The listing builds one solid part. Answer for the finished solid, in the listing's coordinates (mm). Coordinates: 2 decimals unless noted, no trailing zeros. Loops run counter-clockwise (first coordinate to the right, second up) from the corner with the lowest first, then second, coordinate; pieces in that order, holes last. Notation, with made-up numbers: (-9.5, 26.5) -> (28.5, 26.5) arc R20 cw to (28.5, 33.5) -> close; hole circle Ø11 at (88.5, -33). An arc over 180 degrees is marked (long way). Answer in a Markdown table with one row per item.
```python
from build123d import *

# Parameters (mm, degrees)
SKETCH1_R           = 10
SKETCH1_R_2         = 0.5
BOSS_EXTRUDE1_DEPTH = 3


with BuildPart() as part:
    # Sketch1 → Boss-Extrude1 (new body)
    with BuildSketch(Plane.XY):
        Circle(SKETCH1_R)
        with Locations((0, 9)):
            Circle(SKETCH1_R_2, mode=Mode.SUBTRACT)
        Polygon((2, -0.866025404), (3.5, -1.732050808), (5, -0.866025404), (5, 0.866025404), (3.5, 1.732050808), (2, 0.866025404), align=None, mode=Mode.SUBTRACT)
        Polygon((-1.75, 1.267949192), (-0.25, 2.133974596), (-0.25, 3.866025404), (-1.75, 4.732050808), (-3.25, 3.866025404), (-3.25, 2.133974596), align=None, mode=Mode.SUBTRACT)
        Polygon((-1.5, -0.866025404), (0, -1.732050808), (1.5, -0.866025404), (1.5, 0.866025404), (0, 1.732050808), (-1.5, 0.866025404), align=None, mode=Mode.SUBTRACT)
        Polygon((5.5, -0.866025404), (7, -1.732050808), (8.5, -0.866025404), (8.5, 0.866025404), (7, 1.732050808), (5.5, 0.866025404), align=None, mode=Mode.SUBTRACT)
        Polygon((-5.5, 0.866025404), (-5.5, -0.866025404), (-7, -1.732050808), (-8.5, -0.866025404), (-8.5, 0.866025404), (-7, 1.732050808), align=None, mode=Mode.SUBTRACT)
        Polygon((-2, 0.866025404), (-2, -0.866025404), (-3.5, -1.732050808), (-5, -0.866025404), (-5, 0.866025404), (-3.5, 1.732050808), align=None, mode=Mode.SUBTRACT)
        Polygon((1.75, 1.267949192), (3.25, 2.133974596), (3.25, 3.866025404), (1.75, 4.732050808), (0.25, 3.866025404), (0.25, 2.133974596), align=None, mode=Mode.SUBTRACT)
        Polygon((5.25, 1.267949192), (6.75, 2.133974596), (6.75, 3.866025404), (5.25, 4.732050808), (3.75, 3.866025404), (3.75, 2.133974596), align=None, mode=Mode.SUBTRACT)
        Polygon((-0.25, -2.133974596), (-1.75, -1.267949192), (-3.25, -2.133974596), (-3.25, -3.866025404), (-1.75, -4.732050808), (-0.25, -3.866025404), align=None, mode=Mode.SUBTRACT)
        Polygon((3.25, -2.133974596), (1.75, -1.267949192), (0.25, -2.133974596), (0.25, -3.866025404), (1.75, -4.732050808), (3.25, -3.866025404), align=None, mode=Mode.SUBTRACT)
        Polygon((-3.75, -2.133974596), (-5.25, -1.267949192), (-6.75, -2.133974596), (-6.75, -3.866025404), (-5.25, -4.732050808), (-3.75, -3.866025404), align=None, mode=Mode.SUBTRACT)
    extrude(amount=BOSS_EXTRUDE1_DEPTH)


solid = part.part
```
Item 1: Flat-ended cylindrical pins translate along their axes: pin 1 Ø1.4 at (y, z) = (0.5, 1.5) entering from +X; pin 2 Ø1.5 at (x, z) = (-5.5, 2) entering from -Y; pin 3 Ø0.9 at (y, z) = (3, 2) entering from +X; pin 4 Ø0.5 at (y, z) = (3, 2) entering from +X. Find the tip coordinate at first contact, or state that the pin passes through.
Findings below:
| item | result |
|---|---|
| pin 1 | stops at x = 10 |
| pin 2 | stops at y = -8.8 |
| pin 3 | stops at x = 9.67 |
| pin 4 | stops at x = 9.61 |
Item 2: A cutting plane is placed at D-D, the plane y = 9. Determine the outline of the cut face in (x, z), plus the area to 3 significant figures.
Findings below:
| item | result |
|---|---|
| outline | (-4.36, 0) -> (-0.5, 0) -> (-0.5, 3) -> (-4.36, 3) -> close; (0.5, 0) -> (4.36, 0) -> (4.36, 3) -> (0.5, 3) -> close |
| area | 23.2 mm2 |
Item 3: A cutting plane is placed at A-A, the plane y = 0. Determine the outline of the cut face in (x, z).
Findings below:
| item | result |
|---|---|
| outline | (-10, 0) -> (-8.5, 0) -> (-8.5, 3) -> (-10, 3) -> close; (-5.5, 0) -> (-5, 0) -> (-5, 3) -> (-5.5, 3) -> close; (-2, 0) -> (-1.5, 0) -> (-1.5, 3) -> (-2, 3) -> close; (1.5, 0) -> (2, 0) -> (2, 3) -> (1.5, 3) -> close; (5, 0) -> (5.5, 0) -> (5.5, 3) -> (5, 3) -> close; (8.5, 0) -> (10, 0) -> (10, 3) -> (8.5, 3) -> close |
Item 4: A cutting plane is placed at B-B, the plane x = -4.25. Determine the outline of the cut face in (y, z), plus the area to 3 significant figures.
Findings below:
| item | result |
|---|---|
| outline | (-9.05, 0) -> (-4.15, 0) -> (-4.15, 3) -> (-9.05, 3) -> close; (-1.85, 0) -> (-1.3, 0) -> (-1.3, 3) -> (-1.85, 3) -> close; (1.3, 0) -> (9.05, 0) -> (9.05, 3) -> (1.3, 3) -> close |
| area | 39.6 mm2 |
Item 5: Find the intervals of material crossed by probe 1 along Y at (x, z) = (-4.75, 0.1); probe 2 along X at (y, z) = (-4, 1.6); probe 3 along Y at (x, z) = (-3, 0.5), in increasing order.
Findings below:
| item | result |
|---|---|
| probe 1 | y = -8.8 to -4.44, -1.56 to -1.01, 1.01 to 8.8 |
| probe 2 | x = -9.17 to -6.52, -3.98 to -3.02, -0.48 to 0.48, 3.02 to 9.17 |
| probe 3 | y = -9.54 to -4.01, -1.99 to -1.44, 1.44 to 1.99, 4.01 to 9.54 |
Item 6: A cutting plane is placed at C-C, the plane y = 2.5. Determine the outline of the cut face in (x, z).
Findings below:
| item | result |
|---|---|
| outline | (-9.68, 0) -> (-3.25, 0) -> (-3.25, 3) -> (-9.68, 3) -> close; (-0.25, 0) -> (0.25, 0) -> (0.25, 3) -> (-0.25, 3) -> close; (3.25, 0) -> (3.75, 0) -> (3.75, 3) -> (3.25, 3) -> close; (6.75, 0) -> (9.68, 0) -> (9.68, 3) -> (6.75, 3) -> close |
Item 7: Determine the mould class of faces 1 (the face through (0, -2, 3)), 2 (the face through (5, 0, 1)) for opening direction Y: +Y half, -Y half, draft (parallel to the pull), parting line (faces both ways), or undercut.
Findings below:
| item | result |
|---|---|
| face 1 | draft |
| face 2 | undercut |
